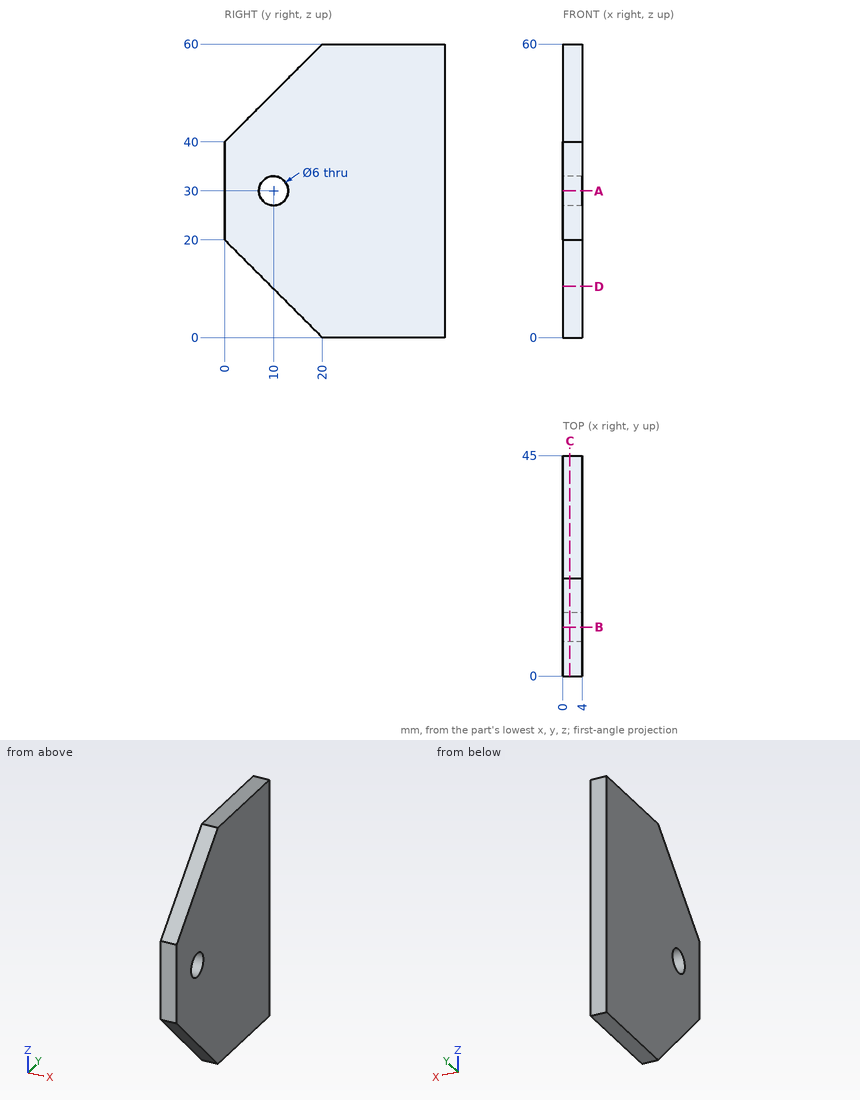
Print and shaded views of the part. All mm, measured from the part's lowest x, y and z. Give positions to 0.01 mm unless a question says otherwise; leave off trailing zeros. Loops run counter-clockwise (first coordinate to the right, second up) from the corner with the lowest first, then second, coordinate; pieces in that order, holes last. Notation, with made-up numbers: (-19.75, 59.5) - (28.25, 59.5) arc R23 cw to (28.25, 95.5) - close; hole circle Ø2 at (41, 72.5). An arc over 180 degrees is marked (long way). Use a Markdown table: item, result.
(1) Drop flat-ended pins along their axis: pin 1 Ø1.5 at (x, y) = (1.5, 9) entering from +Z; pin 2 Ø2 at (x, y) = (3, 15.5) entering from +Z; pin 3 Ø5 at (y, z) = (10, 30) entering from +X. Give the stop position or say it passes through.
Taken from the geometry:
| item | result |
|---|---|
| pin 1 | z = 49.75 |
| pin 2 | z = 56.5 |
| pin 3 | through |
(2) Wall check: line 1 along Y through (x, z) = (2.6, 30); line 2 along Z through (x, y) = (3.1, 10); line 3 along Y through (x, z) = (0.5, 51). Give the ranges that are in metal, low to high.
Taken from the geometry:
| item | result |
|---|---|
| line 1 | 0 to 7, 13 to 45 |
| line 2 | 10 to 27, 33 to 50 |
| line 3 | 11 to 45 |
(3) Band-saw the part on A-A (z = 30). Give the cut face in (x, y).
Taken from the geometry:
| item | result |
|---|---|
| outline | (0, 0) - (4, 0) - (4, 7) - (0, 7) - close; (0, 13) - (4, 13) - (4, 45) - (0, 45) - close |
(4) Band-saw the part on D-D (z = 10.5). Give the cut face in (x, y).
Taken from the geometry:
| item | result |
|---|---|
| outline | (0, 9.5) - (4, 9.5) - (4, 45) - (0, 45) - close |
(5) Band-saw the part on B-B (y = 10). Give the cut face in (x, z).
Taken from the geometry:
| item | result |
|---|---|
| outline | (0, 10) - (4, 10) - (4, 27) - (0, 27) - close; (0, 33) - (4, 33) - (4, 50) - (0, 50) - close |
(6) Band-saw the part on C-C (x = 1.45). Give the cut face in (y, z).
Taken from the geometry:
| item | result |
|---|---|
| outline | (0, 20) - (20, 0) - (45, 0) - (45, 60) - (20, 60) - (0, 40) - close; hole circle Ø6 at (10, 30) |
